Could you check a few things on this model? Use its own coordinates, in mm. Round coordinates to 2 decimals unless told otherwise and drop trailing zeros. Loops run counter-clockwise (first coordinate to the right, second up) from the corner with the lowest first, then second, coordinate; pieces in that order, holes last. Notation, with made-up numbers: (32.25, -33) -> (63.25, -33) arc R25 cw to (63.25, -2) -> close; hole circle Ø4 at (66.5, 44.25). An arc over 180 degrees is marked (long way). One line per item, written item: value.
Autodesk Inventor part; units mm, degrees
ref_plane "YZ Plane" through (0, 0, 0) normal (1, 0, 0) x (0, 1, 0)
ref_plane "XZ Plane" through (0, 0, 0) normal (0, 1, 0) x (-1, 0, 0)
ref_plane "XY Plane" through (0, 0, 0) normal (0, 0, 1) x (1, 0, 0)
sketch "Sketch1" plane through (0, 0, 0) normal (0, 0, 1) x (1, 0, 0)
  circle A0 centre (-100.7807, -75.4427) radius 1.73
  circle A1 centre (-79.9441, -63.4127) radius 1.73
  circle A2 centre (79.9441, -63.4127) radius 1.73
  circle A3 centre (115.7257, -49.5573) radius 1.73
  circle A4 centre (94.8891, -37.5273) radius 1.73
  circle A5 centre (100.7807, -75.4427) radius 1.73
  circle A6 centre (-14.945, 125) radius 1.73
  circle A7 centre (-14.945, 100.94) radius 1.73
  circle A8 centre (14.945, 125) radius 1.73
  line L0 (10, 182.5) -> (10, 187.5)
  line L1 (10, 187.5) -> (0, 187.5)
  line L2 (50, 182.5) -> (10, 182.5)
  circle A9 centre (-94.8891, -37.5273) radius 1.73
  circle A10 centre (-115.7257, -49.5573) radius 1.73
  circle A11 centre (0, 0) radius 200
  circle A12 centre (14.945, 100.94) radius 1.73
  line L3 (0, 152.5) -> (50, 152.5)
  line L4 (50, 152.5) -> (50, 182.5)
  line L5 (0, 152.5) -> (-50, 152.5)
  line L6 (-10, 187.5) -> (0, 187.5)
  line L7 (-10, 182.5) -> (-10, 187.5)
  line L8 (-50, 182.5) -> (-10, 182.5)
  line L9 (-50, 152.5) -> (-50, 182.5)
  circle A13 centre (0, 0) radius 200
  line L10 (-163.0496, -82.5897) -> (-167.3798, -85.0897)
  line L11 (-167.3798, -85.0897) -> (-162.3798, -93.75)
  line L12 (-183.0496, -47.9487) -> (-163.0496, -82.5897)
  line L13 (-132.0689, -76.25) -> (-157.0689, -32.9487)
  line L14 (-157.0689, -32.9487) -> (-183.0496, -47.9487)
  line L15 (-132.0689, -76.25) -> (-107.0689, -119.5513)
  line L16 (-157.3798, -102.4103) -> (-162.3798, -93.75)
  line L17 (-153.0496, -99.9103) -> (-157.3798, -102.4103)
  line L18 (-133.0496, -134.5513) -> (-153.0496, -99.9103)
  line L19 (-107.0689, -119.5513) -> (-133.0496, -134.5513)
  circle A14 centre (0, 0) radius 200
  line L20 (153.0496, -99.9103) -> (157.3798, -102.4103)
  line L21 (157.3798, -102.4103) -> (162.3798, -93.75)
  line L22 (133.0496, -134.5513) -> (153.0496, -99.9103)
  line L23 (132.0689, -76.25) -> (107.0689, -119.5513)
  line L24 (107.0689, -119.5513) -> (133.0496, -134.5513)
  line L25 (132.0689, -76.25) -> (157.0689, -32.9487)
  line L26 (167.3798, -85.0897) -> (162.3798, -93.75)
  line L27 (163.0496, -82.5897) -> (167.3798, -85.0897)
  line L28 (183.0496, -47.9487) -> (163.0496, -82.5897)
  line L29 (157.0689, -32.9487) -> (183.0496, -47.9487)
  dimension "d4" = 40
  dimension "d5" = 3.46
  dimension "d6" = 360
  dimension "d7" = 50
  dimension "d8" = 360
extrude "Extrusion1" add sketch "Sketch1" along normal blind 5
sketch "Sketch2" plane through (0, 0, 5) normal (0, 0, 1) x (1, 0, 0)
  circle A0 centre (0, 0) radius 195 construction
  line L0 (0, 195) -> (10, 195)
  line L1 (10, 195) -> (10, 190)
  line L2 (10, 190) -> (0, 190)
  circle A1 centre (0, 0) radius 195 construction
  line L3 (0, 195) -> (-10, 195)
  line L4 (-10, 195) -> (-10, 190)
  line L5 (-10, 190) -> (0, 190)
  circle A2 centre (0, 0) radius 195 construction
  line L6 (97.5, 168.875) -> (106.1603, 163.875)
  line L7 (106.1603, 163.875) -> (103.6603, 159.5448)
  line L8 (103.6603, 159.5448) -> (95, 164.5448)
  circle A3 centre (0, 0) radius 195 construction
  line L9 (97.5, 168.875) -> (88.8397, 173.875)
  line L10 (88.8397, 173.875) -> (86.3397, 169.5448)
  line L11 (86.3397, 169.5448) -> (95, 164.5448)
  circle A4 centre (0, 0) radius 195 construction
  line L12 (168.875, 97.5) -> (173.875, 88.8397)
  line L13 (173.875, 88.8397) -> (169.5448, 86.3397)
  line L14 (169.5448, 86.3397) -> (164.5448, 95)
  circle A5 centre (0, 0) radius 195 construction
  line L15 (168.875, 97.5) -> (163.875, 106.1603)
  line L16 (163.875, 106.1603) -> (159.5448, 103.6603)
  line L17 (159.5448, 103.6603) -> (164.5448, 95)
  circle A6 centre (0, 0) radius 195 construction
  line L18 (195, 0) -> (195, -10)
  line L19 (195, -10) -> (190, -10)
  line L20 (190, -10) -> (190, 0)
  circle A7 centre (0, 0) radius 195 construction
  line L21 (195, 0) -> (195, 10)
  line L22 (195, 10) -> (190, 10)
  line L23 (190, 10) -> (190, 0)
  circle A8 centre (0, 0) radius 195 construction
  line L24 (168.875, -97.5) -> (163.875, -106.1603)
  line L25 (163.875, -106.1603) -> (159.5448, -103.6603)
  line L26 (159.5448, -103.6603) -> (164.5448, -95)
  circle A9 centre (0, 0) radius 195 construction
  line L27 (168.875, -97.5) -> (173.875, -88.8397)
  line L28 (173.875, -88.8397) -> (169.5448, -86.3397)
  line L29 (169.5448, -86.3397) -> (164.5448, -95)
  circle A10 centre (0, 0) radius 195 construction
  line L30 (97.5, -168.875) -> (88.8397, -173.875)
  line L31 (88.8397, -173.875) -> (86.3397, -169.5448)
  line L32 (86.3397, -169.5448) -> (95, -164.5448)
  circle A11 centre (0, 0) radius 195 construction
  line L33 (97.5, -168.875) -> (106.1603, -163.875)
  line L34 (106.1603, -163.875) -> (103.6603, -159.5448)
  line L35 (103.6603, -159.5448) -> (95, -164.5448)
  circle A12 centre (0, 0) radius 195 construction
  line L36 (0, -195) -> (-10, -195)
  line L37 (-10, -195) -> (-10, -190)
  line L38 (-10, -190) -> (0, -190)
  circle A13 centre (0, 0) radius 195 construction
  line L39 (0, -195) -> (10, -195)
  line L40 (10, -195) -> (10, -190)
  line L41 (10, -190) -> (0, -190)
  circle A14 centre (0, 0) radius 195 construction
  line L42 (-97.5, -168.875) -> (-106.1603, -163.875)
  line L43 (-106.1603, -163.875) -> (-103.6603, -159.5448)
  line L44 (-103.6603, -159.5448) -> (-95, -164.5448)
  circle A15 centre (0, 0) radius 195 construction
  line L45 (-97.5, -168.875) -> (-88.8397, -173.875)
  line L46 (-88.8397, -173.875) -> (-86.3397, -169.5448)
  line L47 (-86.3397, -169.5448) -> (-95, -164.5448)
  circle A16 centre (0, 0) radius 195 construction
  line L48 (-168.875, -97.5) -> (-173.875, -88.8397)
  line L49 (-173.875, -88.8397) -> (-169.5448, -86.3397)
  line L50 (-169.5448, -86.3397) -> (-164.5448, -95)
  circle A17 centre (0, 0) radius 195 construction
  line L51 (-168.875, -97.5) -> (-163.875, -106.1603)
  line L52 (-163.875, -106.1603) -> (-159.5448, -103.6603)
  line L53 (-159.5448, -103.6603) -> (-164.5448, -95)
  circle A18 centre (0, 0) radius 195 construction
  line L54 (-195, 0) -> (-195, 10)
  line L55 (-195, 10) -> (-190, 10)
  line L56 (-190, 10) -> (-190, 0)
  circle A19 centre (0, 0) radius 195 construction
  line L57 (-195, 0) -> (-195, -10)
  line L58 (-195, -10) -> (-190, -10)
  line L59 (-190, -10) -> (-190, 0)
  circle A20 centre (0, 0) radius 195 construction
  line L60 (-168.875, 97.5) -> (-163.875, 106.1603)
  line L61 (-163.875, 106.1603) -> (-159.5448, 103.6603)
  line L62 (-159.5448, 103.6603) -> (-164.5448, 95)
  circle A21 centre (0, 0) radius 195 construction
  line L63 (-168.875, 97.5) -> (-173.875, 88.8397)
  line L64 (-173.875, 88.8397) -> (-169.5448, 86.3397)
  line L65 (-169.5448, 86.3397) -> (-164.5448, 95)
  circle A22 centre (0, 0) radius 195 construction
  line L66 (-97.5, 168.875) -> (-88.8397, 173.875)
  line L67 (-88.8397, 173.875) -> (-86.3397, 169.5448)
  line L68 (-86.3397, 169.5448) -> (-95, 164.5448)
  circle A23 centre (0, 0) radius 195 construction
  line L69 (-97.5, 168.875) -> (-106.1603, 163.875)
  line L70 (-106.1603, 163.875) -> (-103.6603, 159.5448)
  line L71 (-103.6603, 159.5448) -> (-95, 164.5448)
  dimension "d11" = 390
  dimension "d12" = 10
  dimension "d13" = 5
  dimension "d16" = 360
extrude "Extrusion2" cut sketch "Sketch2" against normal blind 5 contours L6 L7 L8 L11 L10 L9 | L12 L13 L14 L17 L16 L15 | L18 L19 L20 L23 L22 L21 | L30 L31 L32 L35 L34 L33 | L36 L37 L38 L41 L40 L39 | L42 L43 L44 L47 L46 L45 | L54 L55 L56 L59 L58 L57 | L60 L61 L62 L65 L64 L63 | L66 L67 L68 L71 L70 L69
sketch "Sketch3" plane through (0, 0, 5) normal (0, 0, 1) x (1, 0, 0)
  line L0 (88.8397, 173.875) -> (106.1603, 163.875)
  circle A0 centre (90, 155.8846) radius 1.5
  circle A1 centre (0, 180) radius 1.5
  circle A2 centre (-90, 155.8846) radius 1.5
  circle A3 centre (-155.8846, 90) radius 1.5
  circle A4 centre (-180, 0) radius 1.5
  circle A5 centre (-155.8846, -90) radius 1.5
  circle A6 centre (-90, -155.8846) radius 1.5
  circle A7 centre (0, -180) radius 1.5
  circle A8 centre (90, -155.8846) radius 1.5
  circle A9 centre (155.8846, -90) radius 1.5
  circle A10 centre (180, 0) radius 1.5
  circle A11 centre (155.8846, 90) radius 1.5
  point P0 (0, 0)
  point P1 (0, 0)
  dimension "d21" = 3
  dimension "d24" = 360
extrude "Extrusion3" cut sketch "Sketch3" against normal blind 5 contours A0 | A2 | A3 | A4 | A6 | A7 | A8 | A10 | A11
sketch "Sketch4" plane through (0, 0, 5) normal (0, 0, 1) x (1, 0, 0)
  line L0 (0, 0) -> (100, 0) construction
  circle A0 centre (70.7107, 70.7107) radius 1.5
  circle A1 centre (-70.7107, 70.7107) radius 1.5
  circle A2 centre (-70.7107, -70.7107) radius 1.5
  circle A3 centre (70.7107, -70.7107) radius 1.5
  dimension "d30" = 3
  dimension "d33" = 360
extrude "Extrusion4" cut sketch "Sketch4" against normal blind 5
properties part number "De_final"
(1) Please list where these lines run through material, in increasing order: L1, parallel to Y at x = -6, z = 3.35; L2, parallel to X at y = 6, z = 2.6; L3, parallel to Y at x = 80.5, z = 0.65.
Results below:
L1: y = -199.91 to -195, -190 to 152.5, 187.5 to 199.91
L2: x = -199.91 to -195, -190 to 190, 195 to 199.91
L3: y = -183.08 to -65.05, -61.77 to 183.08
(2) Imagine slicing it at A-A on x = -25.5. Write out the boundary of the cut face in (y, z).
Results below:
outline: (-198.37, 0) -> (152.5, 0) -> (152.5, 5) -> (-198.37, 5) -> close; (182.5, 0) -> (198.37, 0) -> (198.37, 5) -> (182.5, 5) -> close
(3) Imagine slicing it at B-B on z = 3.7. Give the number of separate pieces and of enclosed holes in the cut face, then the cut area to 3 significant figures.
Results below:
separate pieces: 1
enclosed holes: 37
area: 115,000 mm²
(4) We'd pull the mould along X, two halves only. Please class faces 1 (the face through (164.615, 94.879, 2.535)), 2 (the face through (190.764, -60.075, 2.465)), 3 (the face through (-3, 3, 0)): +X half, -X half, draft (parallel to the pull), parting line (faces both ways), or undercut.
Results below:
face 1: undercut
face 2: parting line
face 3: draft
(5) For pin 1 Ø3 at (x, y) = (14.945, 100.94) entering from -Z; pin 2 Ø3 at (x, z) = (79.5, 2) entering from +Y; pin 3 Ø1.5 at (x, z) = (-3.5, 3.5) entering from -Y, each with a flat end and sliding along its axis, tell me the tip position at first contact or that it passes through.
Results below:
pin 1: passes through
pin 2: stops at y = 184.16
pin 3: stops at y = -199.98
